Input: dimensioned drawing with shaded views. Units: mm. Origin: part minimum x, y, z. Give positions to 0.01 mm unless a question says otherwise; leave off trailing zeros. Order: outer loops, then holes, each group sorted by start corner. A loop starts at its lowest first (then second) coordinate and runs counter-clockwise, first axis right, second up. Notation, with made-up numbers: (60.5, 22) - (93.5, 22) arc R11 cw to (93.5, 27) - close; hole circle Ø11 at (68.25, -36). An arc over 180 degrees is marked (long way). Use a Markdown table: item, result.
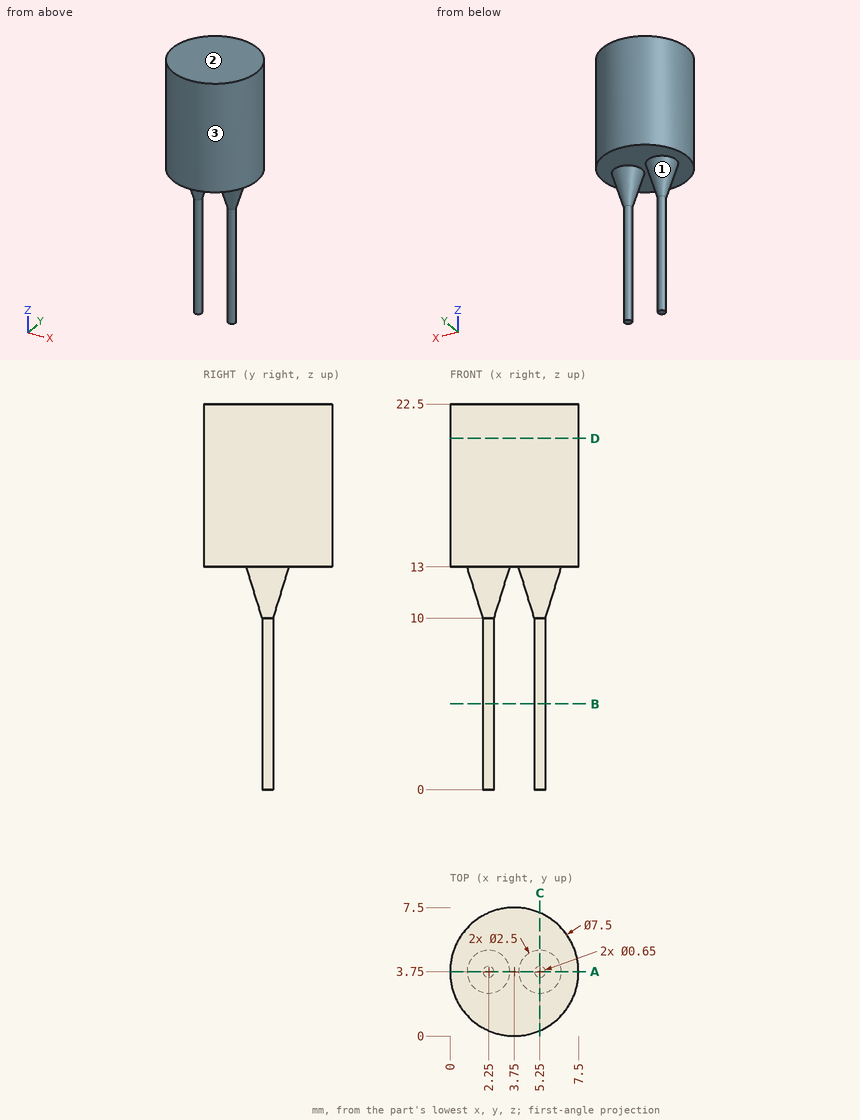
1. Pin query (flat end, axial travel): pin 1 (1 mm diameter, centred on x = 3, z = 20, fed in from +Y); pin 2 (3 mm diameter, centred on y = 2, z = 14.5, fed in from -X); pin 3 (2 mm diameter, centred on y = 3.5, z = 9.5, fed in from -X). Return the tip coordinate at first contact, or that it passes through.
Response:
| item | result |
|---|---|
| pin 1 | stops at y = 7.49 |
| pin 2 | stops at x = 0.01 |
| pin 3 | stops at x = 1.78 |
2. Section query D-D (z = 20.5). Return loops of the section in (x, y).
Response:
| item | result |
|---|---|
| outline | circle Ø7.5 at (3.75, 3.75) |
3. Section query B-B (z = 5). Return loops of the section in (x, y) (3 decimals).
Response:
| item | result |
|---|---|
| outline | circle Ø0.65 at (2.25, 3.75); circle Ø0.65 at (5.25, 3.75) |
4. Mould query, pull axis X, two halves, no side actions, for the marked faces 1, 2 and 3. Classes: pulls with the +X half, pulls with the -X half, needs draft (parallel to the pull), parting line crosses it, or undercut.
Response:
| item | result |
|---|---|
| face 1 | undercut |
| face 2 | needs draft |
| face 3 | parting line crosses it |
5. Section query C-C (x = 5.25). Return loops of the section in (y, z) (3 decimals), then the cut area to 3 significant figures.
Response:
| item | result |
|---|---|
| outline | (0.313, 13) - (2.5, 13) - (3.425, 10) - (3.425, 0) - (4.075, 0) - (4.075, 10) - (5, 13) - (7.187, 13) - (7.187, 22.5) - (0.313, 22.5) - close |
| area | 76.5 mm^2 |
6. Material intervals for line 1 along Z through (x, y) = (6.5, 5.25); line 2 along X through (y, z) = (5, 21.75); line 3 along Y through (x, z) = (5, 3.75), sorted ascending.
Response:
| item | result |
|---|---|
| line 1 | z = 13 to 22.5 |
| line 2 | x = 0.21 to 7.29 |
| line 3 | y = 3.54 to 3.96 |
7. Section query A-A (y = 3.75). Return loops of the section in (x, z) (3 decimals), then the cut area to 3 significant figures.
Response:
| item | result |
|---|---|
| outline | (0, 13) - (1, 13) - (1.925, 10) - (1.925, 0) - (2.575, 0) - (2.575, 10) - (3.5, 13) - (4, 13) - (4.925, 10) - (4.925, 0) - (5.575, 0) - (5.575, 10) - (6.5, 13) - (7.5, 13) - (7.5, 22.5) - (0, 22.5) - close |
| area | 93.7 mm^2 |
